Autodesk Inventor part; units mm, degrees
ref_plane "YZ Plane" through (0, 0, 0) normal (1, 0, 0) x (0, 1, 0)
ref_plane "XZ Plane" through (0, 0, 0) normal (0, 1, 0) x (-1, 0, 0)
ref_plane "XY Plane" through (0, 0, 0) normal (0, 0, 1) x (1, 0, 0)
sketch "スケッチ1" plane through (0, 0, 0) normal (1, 0, 0) x (0, 1, 0)
  circle A0 centre (0, 0) radius 9.75
  dimension "d0" = 19.5
extrude "押し出し1" add sketch "スケッチ1" along normal blind 1.4
sketch "スケッチ2" plane through (1.4, 0, 0) normal (1, 0, 0) x (0, 0, -1)
  circle A0 centre (0, 0) radius 9.75
  line L0 (0, 0) -> (0, -7.5)
  line L1 (0, -7.5) -> (11, -7.5)
  line L2 (11, -7.5) -> (11, 7.5)
  line L3 (11, 7.5) -> (0, 7.5)
  line L4 (0, 7.5) -> (0, 0)
  point P0 (6.23, 7.5)
  point P1 (6.23, -7.5)
  dimension "d3" = 7.5
  dimension "d4" = 11
  dimension "d5" = 15
extrude "押し出し2" add sketch "スケッチ2" against normal blind 1.4 contours A0 L3 L2 L1
sketch "スケッチ4" plane through (1.4, 0, 0) normal (1, 0, 0) x (0, 0, -1)
  line L0 (11, -7.5) -> (6.23, -7.5)
  line L1 (6.23, 7.5) -> (11, 7.5)
  line L2 (11, -7.5) -> (9.5, -7.5)
  line L3 (9.5, -7.5) -> (9.5, 7.5)
  line L4 (9.5, 7.5) -> (11, 7.5)
  line L5 (11, 7.5) -> (11, -7.5)
  point P0 (0, 0)
  dimension "d13" = 1.5
extrude "押し出し4" add sketch "スケッチ4" along normal blind 48
sketch "スケッチ5" plane through (1.4, -7.5, -9.5) normal (0, 0, 1) x (1, 0, 0)
  line L0 (48, 15) -> (48, 0)
  line L1 (48, 15) -> (-1.4, 15)
  line L2 (48, 0) -> (46.5, 0)
  line L3 (46.5, 0) -> (46.5, 15)
  line L4 (46.5, 15) -> (48, 15)
  line L5 (48, 15) -> (48, 0)
  point P0 (-1.4, 7.5)
  dimension "d16" = 1.5
extrude "押し出し5" add sketch "スケッチ5" along normal blind 13.2
sketch "スケッチ6" plane through (0, 0, 0) normal (-1, 0, 0) x (0, 0, 1)
  circle A0 centre (0, 0) radius 1.5
  circle A1 centre (-4, 5) radius 1.5
  circle A2 centre (-4, -5) radius 1.5
  dimension "d19" = 3
  dimension "d20" = 3
  dimension "d21" = 3
extrude "押し出し6" cut sketch "スケッチ6" against normal blind 50
fillet "フィレット1" radius 3 2 edges at (48.65, 7.5, 3.7) (48.65, -7.5, 3.7)
fillet "フィレット2" radius 3 2 edges at (49.4, 0, -11) (0, 0, -11)
fillet "フィレット3" radius 2 2 edges at (1.4, 0, -9.5) (47.9, 0, -9.5)
sketch "スケッチ7" plane through (46.4, 7.5, -11) normal (0, 0, -1) x (-1, 0, 0)
  circle A0 centre (8, -7.5) radius 1.25
  circle A1 centre (32, -7.5) radius 1.25
  point P0 (46.4, -7.5)
  dimension "d27" = 2.5
  dimension "d28" = 2.5
extrude "押し出し7" cut sketch "スケッチ7" against normal blind 13.2
sketch "スケッチ8" plane through (49.4, 0, 0) normal (1, 0, 0) x (0, 0, -1)
  line L0 (11, 1.25) -> (11, -1.25)
  line L1 (11, 0) -> (11, 2)
  line L2 (11, 7.5) -> (11, -7.5)
  line L3 (11, 2) -> (4.5, 2)
  line L4 (4.5, 2) -> (4.5, -2)
  line L5 (4.5, -2) -> (11, -2)
  line L6 (11, -2) -> (11, 0)
  point P0 (0, 0)
  dimension "d31" = 2
  dimension "d32" = 6.5
  dimension "d33" = 4
extrude "押し出し8" cut sketch "スケッチ8" against normal blind 4
sketch "スケッチ9" plane through (49.4, 0, 0) normal (1, 0, 0) x (0, 0, -1)
  line L0 (4.5, 2) -> (4.5, -2)
  circle A0 centre (4.5, 0) radius 2
  point P0 (0, 0)
extrude "押し出し9" cut sketch "スケッチ9" against normal blind 4 contours L0 A0 picked at (3.8804, 0.6667)
thread "ねじ1"
thread "ねじ2"
properties material "アルミニウム"
Input: part model. Units: mm. Frame: model coordinates. A direction names the side the tool comes from. Give positions to 0.01 mm unless a question says otherwise; leave off trailing zeros. Order: outer loops, then holes, each group sorted by start corner. A loop starts at its lowest first (then second) coordinate and runs counter-clockwise, first axis right, second up. Notation, with made-up numbers: (70.25, 42) - (115.25, 42) arc R21 cw to (115.25, 64) - close; hole circle Ø1 at (-9, -10.75). An arc over 180 degrees is marked (long way). Use a Markdown table: item, result.
(1) Section query D-D (y = 0.5). Output: boundary loops of the cut face in (x, z), then the cut area to 3 significant figures.
Computed values:
| item | result |
|---|---|
| outline | (0, -8) arc R3 ccw to (3, -11) - (13.25, -11) - (13.25, -9.5) - (3.4, -9.5) arc R2 cw to (1.4, -7.5) - (1.4, -1.41) - (0, -1.41) - close; (0, 1.41) - (1.4, 1.41) - (1.4, 9.74) - (0, 9.74) - close; (15.55, -11) - (37.25, -11) - (37.25, -9.5) - (15.55, -9.5) - close; (39.55, -11) - (45.4, -11) - (45.4, -9.5) - (39.55, -9.5) - close; (47.9, -2.56) - (49.4, -2.56) - (49.4, -1.41) - (47.9, -1.41) - close; (47.9, 1.41) - (49.4, 1.41) - (49.4, 3.7) - (47.9, 3.7) - close |
| area | 88.3 mm2 |
(2) Line query: line 1 (X direction, y = 3.5, z = 0); line 2 (Y direction, x = 38.4, z = -10.2); line 3 (Y direction, x = 48.2, z = -4). Output: solid intervals per line, ascending. Write a range as from..to.
Computed values:
| item | result |
|---|---|
| line 1 | x = 0..1.4, 47.9..49.4 |
| line 2 | y = -7.5..-1.25, 1.25..7.5 |
| line 3 | y = -7.5..-6.5, -3.5..-1.94, 1.94..3.5, 6.5..7.5 |
(3) Draft query along X for faces 5 (the cylindrical face through (2, 0.11, -8.93)), 6 (the flat face through (0, -2, 1)), 7 (the flat face through (24, 0, -9.5)), 8 (the cylindrical face through (48.7, 0, -2.5)). Return one class per face: released by +X, released by -X, zero draft, split by the parting line, or undercut.
Computed values:
| item | result |
|---|---|
| face 5 | undercut |
| face 6 | released by -X |
| face 7 | undercut |
| face 8 | zero draft |
(4) Section query B-B (z = 0). Output: boundary loops of the cut face in (x, y).
Computed values:
| item | result |
|---|---|
| outline | (0, -9.75) - (1.4, -9.75) - (1.4, -1.5) - (0, -1.5) - close; (0, 1.5) - (1.4, 1.5) - (1.4, 9.75) - (0, 9.75) - close; (47.9, -7.5) - (49.4, -7.5) - (49.4, -1.5) - (47.9, -1.5) - close; (47.9, 1.5) - (49.4, 1.5) - (49.4, 7.5) - (47.9, 7.5) - close |
(5) Section query C-C (y = 5). Output: boundary loops of the cut face in (x, z), then the cut area to 3 significant figures.
Computed values:
| item | result |
|---|---|
| outline | (0, -8) arc R3 ccw to (3, -11) - (46.4, -11) arc R3 ccw to (49.4, -8) - (49.4, -5.5) - (47.9, -5.5) - (47.9, -7.5) arc R2 cw to (45.9, -9.5) - (3.4, -9.5) arc R2 cw to (1.4, -7.5) - (1.4, -5.5) - (0, -5.5) - close; (0, -2.5) - (1.4, -2.5) - (1.4, 8.37) - (0, 8.37) - close; (47.9, -2.5) - (49.4, -2.5) - (49.4, 3.66) - (47.9, 3.66) - close |
| area | 108 mm2 |
(6) Access query for faces 1 (the flat face through (48, -2, -8)), 2 (the cylindrical face through (48.64, 6.6, 2.84)), 3 (the flat face through (49, 0, 3.7)), 4 (the cylindrical face through (0.9, 0.11, -10.14)). Directions: +Z, -Z, +X, -X, +Y, -Y. A direction counts if a zero-diameter tool reaches every point of the face in a straight line with its end or side. Return the directions, or none.
Computed values:
| item | result |
|---|---|
| face 1 | -Z, +X |
| face 2 | +Z, +X, +Y |
| face 3 | +Z, +X, +Y, -Y |
| face 4 | -Z, -X, +Y, -Y |
(7) Pin query (flat end, axial travel): pin 1 (4 mm diameter, centred on x = 6, y = 6.5, fed in from +Z); pin 2 (2.5 mm diameter, centred on y = -5, z = -4, fed in from -X); pin 3 (4.5 mm diameter, centred on x = 47, z = -6.5, fed in from +Y); pin 4 (2 mm diameter, centred on x = 48, z = -7, fed in from -Y). Return the tip coordinate at first contact, or that it passes through.
Computed values:
| item | result |
|---|---|
| pin 1 | stops at z = -9.5 |
| pin 2 | passes through |
| pin 3 | stops at y = 7.5 |
| pin 4 | stops at y = -7.5 |
(8) Section query A-A (x = 38.4). Output: boundary loops of the cut face in (y, z).
Computed values:
| item | result |
|---|---|
| outline | (-7.5, -11) - (-1.25, -11) - (-1.25, -9.5) - (-7.5, -9.5) - close; (1.25, -11) - (7.5, -11) - (7.5, -9.5) - (1.25, -9.5) - close |
